For this review, take the finished solid that the model builds, in its own axes (mm). Round coordinates to 2 decimals unless told otherwise and drop trailing zeros. Order: outer loops, then holes, each group sorted by start corner. A loop starts at its lowest first (then second) coordinate and runs counter-clockwise, first axis right, second up.
from build123d import *

# Parameters (mm, degrees)
SKETCH2_R           = 125
BOSS_EXTRUDE1_DEPTH = 30
FILLET1_R           = 15
SKETCH3_R           = 15
CUT_EXTRUDE1_DEPTH  = 180.30421077
SKETCH6_R           = 30
CUT_EXTRUDE2_DEPTH  = 180.30421077


with BuildPart() as part:
    # Sketch2 → Boss-Extrude1 (new body)
    with BuildSketch(Plane.XY):
        Circle(SKETCH2_R)
    extrude(amount=BOSS_EXTRUDE1_DEPTH)

    # Fillet1
    fillet1_edges = [part.edges().sort_by_distance(p)[0] for p in [
        (-125, 0, 0),
        (-125, 0, 30),
    ]]
    fillet(fillet1_edges, radius=FILLET1_R - 0.0001)  # a hair under: the kernel refuses the full size

    # Sketch3 → Cut-Extrude1 (cut, through all)
    with BuildSketch(Plane.XY.offset(30)):
        Circle(SKETCH3_R)
    extrude(amount=-CUT_EXTRUDE1_DEPTH, mode=Mode.SUBTRACT)

    # Sketch6 → Cut-Extrude2 (cut, through all)
    with BuildSketch(Plane.XY.offset(30)):
        with Locations((0, 60)):
            Circle(SKETCH6_R)
        with Locations((60, 0)):
            Circle(SKETCH6_R)
        with Locations((0, -60)):
            Circle(SKETCH6_R)
        with Locations((-60, 0)):
            Circle(SKETCH6_R)
    extrude(amount=-CUT_EXTRUDE2_DEPTH, mode=Mode.SUBTRACT)


solid = part.part
(1) Draft analysis for pull direction Y (two halves, no side actions). For faces 1 (the face through (-2, -23, 0)), 2 (the face through (-6.503, -89.287, 15.21)), state which applies: pulls with the +Y half, pulls with the -Y half, needs draft (parallel to the pull), parting line crosses it, or undercut.
(2) Add section A-A on x = 0. Count the separate pieces of the cut face and the enclosed holes in it, plus the area to 3 significant figures.
(3) Wall thickness on L1, parallel to Y at x = 0, z = 15; L2, parallel to X at y = 1.5, z = 28.75; L3, parallel to X at y = 6, z = 16: over which ranges is each line inside the solid? List them lowest first.
(4) Add section D-D on z = 6.25. Give the boundary of the cut face in (x, y).
(5) Add section B-B on z = 18.75. Give the boundary of the cut face in (x, y), plus the area to 3 significant figures.
(6) Clearance check with flat-ended pins moving along their axes: P1, Ø2, axis at y = 72, z = 7, coming from the -X side; P2, Ø3, axis at x = -56.5, z = 24, coming from the +Y side; P3, Ø12, axis at x = -26, z = 24, coming from the +Y side. State where each tip first meets the part, or that it passes through.
Here are the results:
1. face 1: needs draft
1. face 2: undercut
2. separate pieces: 4
2. enclosed holes: 0
2. area: 2,810 mm2
3. L1: y = -125 to -90, -30 to -15, 15 to 30, 90 to 125
3. L2: x = -115.99 to -89.96, -30.04 to -14.92, 14.92 to 30.04, 89.96 to 115.99
3. L3: x = -124.82 to -89.39, -30.61 to -13.75, 13.75 to 30.61, 89.39 to 124.82
4. outline: circle Ø244.37 at (0, 0); hole circle Ø60 at (-60, 0); hole circle Ø60 at (0, -60); hole circle Ø60 at (0, 60); hole circle Ø30 at (0, 0); hole circle Ø60 at (60, 0)
5. outline: circle Ø249.05 at (0, 0); hole circle Ø60 at (-60, 0); hole circle Ø60 at (0, -60); hole circle Ø60 at (0, 60); hole circle Ø30 at (0, 0); hole circle Ø60 at (60, 0)
5. area: 36,700 mm2
6. P1: stops at x = -100.36
6. P2: stops at y = 109.51
6. P3: stops at y = 122.37
